Geometry check sheet. Reference: drawing and pictorial views, mm from the part's lowest x, y, z. A direction names the side the tool comes from. Round coordinates to 2 decimals unless told otherwise and drop trailing zeros. Order: outer loops, then holes, each group sorted by start corner. A loop starts at its lowest first (then second) coordinate and runs counter-clockwise, first axis right, second up.
(1) Sectioned sample at D-D (x = 8.5). Record the boundary of the cut face in (y, z).
(2) Set-up check for the marked faces 1 and 2: record each of +Z, -Z, +X, -X, +Y, -Y from which the full face is reachable in a straight line by a thin tool's end or side.
(3) Release check for a two-part mould opening along Y. For the marked faces 3, 4 and 5 record: +Y half, -Y half, draft (parallel to the pull), parting line (faces both ways), or undercut.
(4) Go/stop test with flat-tipped pins: pin 1 (1.6 mm diameter, centred on x = 9.5, z = 0.5, fed in from +Y); pin 2 (1.5 mm diameter, centred on y = 15, z = 12.5, fed in from +X); pin 3 (4 mm diameter, centred on x = 10.5, y = 10.5, fed in from +Z); pin 4 (4.5 mm diameter, centred on x = 18.75, y = 17.75, fed in from +Z). Record where each tip stops, or that it passes through.
(5) Sectioned sample at A-A (z = 10). Give the number of separate pieces and of enclosed holes in the cut face, plus the area to 3 significant figures.
(6) Material ranges on line 1 along X through (y, z) = (17.75, 4); line 2 along Y through (x, z) = (46, 27); line 3 along X through (y, z) = (11, 22.5) (1 decimal), recorded low to high.
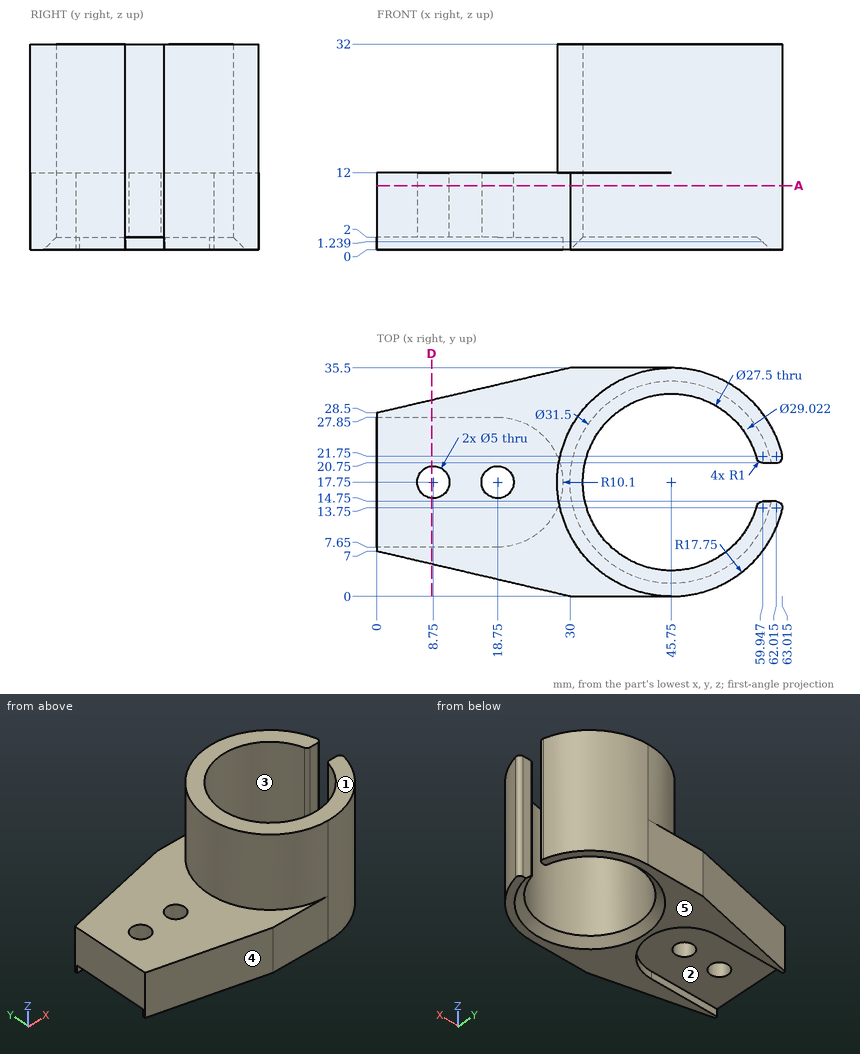
Answer below:
1. outline: (5.02, 0) - (7.65, 0) - (7.65, 2) - (15.26, 2) - (15.26, 12) - (5.02, 12) - close; (20.24, 2) - (27.85, 2) - (27.85, 0) - (30.48, 0) - (30.48, 12) - (20.24, 12) - close
2. face 1: +Z, +X, -X, +Y, -Y
2. face 2: -Z, -X
3. face 3: undercut
3. face 4: -Y half
3. face 5: draft
4. pin 1: stops at y = 30.9
4. pin 2: stops at x = 62.88
4. pin 3: stops at z = 12
4. pin 4: passes through
5. separate pieces: 1
5. enclosed holes: 2
5. area: 1,250 mm2
6. line 1: x = 0 to 6.25, 11.25 to 16.25, 21.25 to 32
6. line 2: y = 0 to 4, 31.5 to 35.5
6. line 3: x = 29.3 to 33.8, 57.7 to 62.2
